Geometry check sheet. Reference: the model listing, model coordinates, mm. A direction names the side the tool comes from. Round coordinates to 2 decimals unless told otherwise and drop trailing zeros. Order: outer loops, then holes, each group sorted by start corner. A loop starts at its lowest first (then second) coordinate and runs counter-clockwise, first axis right, second up.
(1) Set-up check for faces 1 (the face through (-15, -7, -25)), 2 (the face through (0, 20, -25)), 3 (the face through (15, -8, -25)): record each of +Z, -Z, +X, -X, +Y, -Y from which the full face is reachable in a straight line by a thin tool's end or side.
(2) Cross-section at B-B on x = -7.5. Enter the section's corners in (y, z).
(3) Gauge pin test, flat ends, axial feed: P1, Ø6, axis at y = 24, z = 80, coming from the -X side; P2, Ø8, axis at x = -3.5, z = 96.5, coming from the -Y side; P3, Ø24, axis at x = 5, z = -24, coming from the -Y side. Record the tip position at first contact, or that the pin passes through.
(4) Cross-section at D-D on z = 32. Enter the section's corners in (x, y).
(5) Thickness scan on L1, parallel to Z at x = 7.25, y = 0; L2, parallel to X at y = 15.5, z = -34; L3, parallel to Y at x = -9, z = -16. Record the ranges inside material, lowest first.
(6) Cross-section at A-A on y = 0. Enter the section's corners in (x, z).
(7) Draft check along Z on faces 4 (the face through (0, -25, -25)), 5 (the face through (0.21, -0.65, -18.75)), 6 (the face through (0, 0, 150)). Enter one of: pulls with the +Z half, pulls with the -Z half, needs draft (parallel to the pull), parting line crosses it, or undercut.
(8) Cross-section at C-C on y = -10. Enter the section's corners in (x, z).
from build123d import *

# Parameters (mm, degrees)
F0_W          = 30
F0_H          = 150
F2_W          = 30
F2_H          = 100
F3_DEPTH      = 20
F3_DEPTH_BACK = 25
F5_D          = 10


with BuildPart() as f1:
    # F0 (on Front) → F1 (revolve)
    with BuildSketch(Plane.XZ):
        with Locations((15, 75)):
            Rectangle(F0_W, F0_H)
    revolve(axis=Axis((0, 0, 75), (0, 0, 1)))

    # F2 (on Front) → F3 (join, two sides)
    with BuildSketch(Plane.XZ) as f3_sk:
        Rectangle(F2_W, F2_H)
    extrude(amount=-F3_DEPTH)
    extrude(f3_sk.sketch, amount=F3_DEPTH_BACK)

    # F5 (through all)
    with Locations(Plane(origin=(-15, 0, 0), x_dir=(0, -1, 0), z_dir=(-1, 0, 0))):
        with Locations((0, -23.7088240683)):
            Hole(F5_D / 2)


solid = f1.part
Found:
1. face 1: -Z, -X, +Y, -Y
1. face 2: -Z, +X, -X, +Y
1. face 3: -Z, +X, +Y, -Y
2. outline: (-29.05, 0) - (-25, 0) - (-25, -50) - (20, -50) - (20, 0) - (29.05, 0) - (29.05, 150) - (-29.05, 150) - close; hole circle Ø10 at (0, -23.71)
3. P1: stops at x = -21.42
3. P2: stops at y = -30
3. P3: stops at y = -25
4. outline: circle Ø60 at (0, 0)
5. L1: z = -50 to -28.71, -18.71 to 150
5. L2: x = -15 to 15
5. L3: y = -25 to 20
6. outline: (-30, 0) - (-15, 0) - (-15, -18.71) - (15, -18.71) - (15, 0) - (30, 0) - (30, 150) - (-30, 150) - close; (-15, -50) - (15, -50) - (15, -28.71) - (-15, -28.71) - close
7. face 4: needs draft
7. face 5: undercut
7. face 6: pulls with the +Z half
8. outline: (-28.28, 0) - (-15, 0) - (-15, -50) - (15, -50) - (15, 0) - (28.28, 0) - (28.28, 150) - (-28.28, 150) - close
